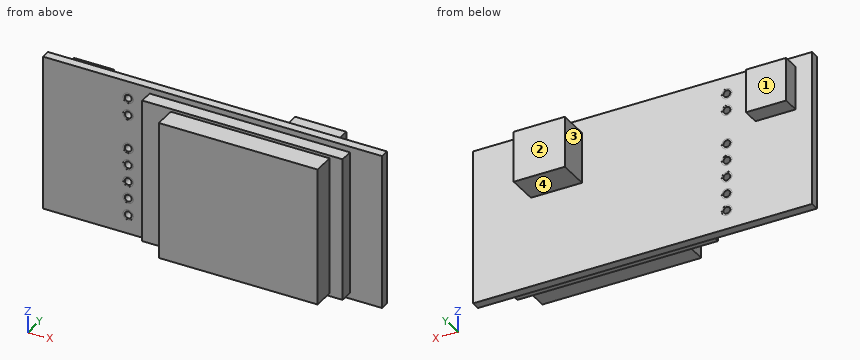
from build123d import *

# Parameters (mm, degrees)
SKETCH1_W           = 49.75
SKETCH1_H           = 22.8
BOSS_EXTRUDE1_DEPTH = 1.3
SKETCH2_W           = 7.5
SKETCH2_H           = 7.5
BOSS_EXTRUDE2_DEPTH = 4.5
SKETCH3_W           = 5.9
SKETCH3_H           = 6.4
BOSS_EXTRUDE3_DEPTH = 2.5
SKETCH4_W           = 29.4
SKETCH4_H           = 21.1
BOSS_EXTRUDE4_DEPTH = 1.95
SKETCH5_W           = 23.3
SKETCH5_H           = 20.25
BOSS_EXTRUDE5_DEPTH = 3.15
CUT_EXTRUDE1_REACH  = 29.971
SKETCH6_R           = 0.5
SKETCH7_R           = 0.75
CUT_EXTRUDE2_DEPTH  = 0.01
CUT_EXTRUDE3_START  = -0.01
SKETCH8_R           = 0.75
CUT_EXTRUDE3_DEPTH  = 0.01


with BuildPart() as part:
    # Sketch1 → Boss-Extrude1 (new body)
    with BuildSketch(Plane(origin=(0, 0, 0), x_dir=(1, 0, 0), z_dir=(0, 1, 0))):
        Rectangle(SKETCH1_W, SKETCH1_H)
    extrude(amount=BOSS_EXTRUDE1_DEPTH)

    # Sketch2 → Boss-Extrude2 (add)
    with BuildSketch(Plane(origin=(0, 1.3, 0), x_dir=(1, 0, 0), z_dir=(0, 1, 0))):
        with Locations((12.625, -5.65)):
            Rectangle(SKETCH2_W, SKETCH2_H)
    extrude(amount=BOSS_EXTRUDE2_DEPTH)

    # Sketch3 → Boss-Extrude3 (add)
    with BuildSketch(Plane(origin=(0, 1.3, 0), x_dir=(1, 0, 0), z_dir=(0, 1, 0))):
        with Locations((-19.525, -6.7)):
            Rectangle(SKETCH3_W, SKETCH3_H)
    extrude(amount=BOSS_EXTRUDE3_DEPTH)

    # Sketch4 → Boss-Extrude4 (add)
    with BuildSketch(Plane.XZ):
        with Locations((5.475, 0)):
            Rectangle(SKETCH4_W, SKETCH4_H)
    extrude(amount=BOSS_EXTRUDE4_DEPTH)

    # Sketch5 → Boss-Extrude5 (add)
    with BuildSketch(Plane.XZ.offset(1.95)):
        with Locations((6.625, 0)):
            Rectangle(SKETCH5_W, SKETCH5_H)
    extrude(amount=BOSS_EXTRUDE5_DEPTH)

    # Sketch6 → Cut-Extrude1 (cut, up to next)
    with BuildSketch(Plane.XZ, mode=Mode.PRIVATE) as cut_extrude1_sk1:
        with Locations(Location((-12.375, 8.9, 0), (0, 0, 270))):
            Circle(SKETCH6_R)
    cut_extrude1_tool1 = extrude(cut_extrude1_sk1.sketch, amount=-CUT_EXTRUDE1_REACH, mode=Mode.PRIVATE) & part.part
    # Sketch6 → Cut-Extrude1 (cut, up to next)
    with BuildSketch(Plane.XZ, mode=Mode.PRIVATE) as cut_extrude1_sk2:
        with Locations(Location((-12.375, 6.4, 0), (0, 0, 270))):
            Circle(SKETCH6_R)
    cut_extrude1_tool2 = extrude(cut_extrude1_sk2.sketch, amount=-CUT_EXTRUDE1_REACH, mode=Mode.PRIVATE) & part.part
    # Sketch6 → Cut-Extrude1 (cut, up to next)
    with BuildSketch(Plane.XZ, mode=Mode.PRIVATE) as cut_extrude1_sk3:
        with Locations(Location((-12.375, 1.4, 0), (0, 0, 270))):
            Circle(SKETCH6_R)
    cut_extrude1_tool3 = extrude(cut_extrude1_sk3.sketch, amount=-CUT_EXTRUDE1_REACH, mode=Mode.PRIVATE) & part.part
    # Sketch6 → Cut-Extrude1 (cut, up to next)
    with BuildSketch(Plane.XZ, mode=Mode.PRIVATE) as cut_extrude1_sk4:
        with Locations(Location((-12.375, -1.1, 0), (0, 0, 270))):
            Circle(SKETCH6_R)
    cut_extrude1_tool4 = extrude(cut_extrude1_sk4.sketch, amount=-CUT_EXTRUDE1_REACH, mode=Mode.PRIVATE) & part.part
    # Sketch6 → Cut-Extrude1 (cut, up to next)
    with BuildSketch(Plane.XZ, mode=Mode.PRIVATE) as cut_extrude1_sk5:
        with Locations(Location((-12.375, -3.6, 0), (0, 0, 270))):
            Circle(SKETCH6_R)
    cut_extrude1_tool5 = extrude(cut_extrude1_sk5.sketch, amount=-CUT_EXTRUDE1_REACH, mode=Mode.PRIVATE) & part.part
    # Sketch6 → Cut-Extrude1 (cut, up to next)
    with BuildSketch(Plane.XZ, mode=Mode.PRIVATE) as cut_extrude1_sk6:
        with Locations(Location((-12.375, -6.1, 0), (0, 0, 270))):
            Circle(SKETCH6_R)
    cut_extrude1_tool6 = extrude(cut_extrude1_sk6.sketch, amount=-CUT_EXTRUDE1_REACH, mode=Mode.PRIVATE) & part.part
    # Sketch6 → Cut-Extrude1 (cut, up to next)
    with BuildSketch(Plane.XZ, mode=Mode.PRIVATE) as cut_extrude1_sk7:
        with Locations(Location((-12.375, -8.6, 0), (0, 0, 270))):
            Circle(SKETCH6_R)
    cut_extrude1_tool7 = extrude(cut_extrude1_sk7.sketch, amount=-CUT_EXTRUDE1_REACH, mode=Mode.PRIVATE) & part.part
    add(cut_extrude1_tool1.solids().sort_by_distance((-12.375, 0, 8.9))[0], mode=Mode.SUBTRACT)
    add(cut_extrude1_tool2.solids().sort_by_distance((-12.375, 0, 6.4))[0], mode=Mode.SUBTRACT)
    add(cut_extrude1_tool3.solids().sort_by_distance((-12.375, 0, 1.4))[0], mode=Mode.SUBTRACT)
    add(cut_extrude1_tool4.solids().sort_by_distance((-12.375, 0, -1.1))[0], mode=Mode.SUBTRACT)
    add(cut_extrude1_tool5.solids().sort_by_distance((-12.375, 0, -3.6))[0], mode=Mode.SUBTRACT)
    add(cut_extrude1_tool6.solids().sort_by_distance((-12.375, 0, -6.1))[0], mode=Mode.SUBTRACT)
    add(cut_extrude1_tool7.solids().sort_by_distance((-12.375, 0, -8.6))[0], mode=Mode.SUBTRACT)

    # Sketch7 → Cut-Extrude2 (cut)
    with BuildSketch(Plane.XZ):
        with Locations(Location((-12.375, 8.9, 0), (0, 0, 270))):
            Circle(SKETCH7_R)
        with Locations(Location((-12.375, 6.4, 0), (0, 0, 270))):
            Circle(SKETCH7_R)
        with Locations(Location((-12.375, 1.4, 0), (0, 0, 270))):
            Circle(SKETCH7_R)
        with Locations(Location((-12.375, -1.1, 0), (0, 0, 270))):
            Circle(SKETCH7_R)
        with Locations(Location((-12.375, -3.6, 0), (0, 0, 270))):
            Circle(SKETCH7_R)
        with Locations(Location((-12.375, -6.1, 0), (0, 0, 270))):
            Circle(SKETCH7_R)
        with Locations(Location((-12.375, -8.6, 0), (0, 0, 270))):
            Circle(SKETCH7_R)
    extrude(amount=-CUT_EXTRUDE2_DEPTH, mode=Mode.SUBTRACT)

    # Sketch8 → Cut-Extrude3 (cut)
    with BuildSketch(Plane(origin=(0, 1.3, 0), x_dir=(1, 0, 0), z_dir=(0, 1, 0)).offset(CUT_EXTRUDE3_START)):
        with Locations(Location((-12.375, 8.6, 0), (0, 0, 90))):
            Circle(SKETCH8_R)
        with Locations(Location((-12.375, 6.1, 0), (0, 0, 90))):
            Circle(SKETCH8_R)
        with Locations(Location((-12.375, 3.6, 0), (0, 0, 90))):
            Circle(SKETCH8_R)
        with Locations(Location((-12.375, 1.1, 0), (0, 0, 90))):
            Circle(SKETCH8_R)
        with Locations(Location((-12.375, -1.4, 0), (0, 0, 90))):
            Circle(SKETCH8_R)
        with Locations(Location((-12.375, -6.4, 0), (0, 0, 90))):
            Circle(SKETCH8_R)
        with Locations(Location((-12.375, -8.9, 0), (0, 0, 90))):
            Circle(SKETCH8_R)
    extrude(amount=CUT_EXTRUDE3_DEPTH, mode=Mode.SUBTRACT)


solid = part.part
Geometry: final body of the model. Coordinates: model frame, mm. Face numbers are marked on the shaded views. A direction names the side the tool comes from. Give positions to 0.01 mm unless a question says otherwise; leave off trailing zeros. Write each loop counter-clockwise with the first axis right and the second up, starting at its lowest first coordinate (ties: lowest second). Pieces come first, ordered by that corner, then holes.
(1) Cut plane B-B, the plane y = 3.25. Return loops of the section in (x, z) (3 decimals), then the cut area to 3 significant figures.
(2) First-contact query: P1, Ø1.4, axis at x = -12.375, z = -1.1, coming from the +Y side; P2, Ø0.8, axis at x = -12, z = -6, coming from the -Y side; P3, Ø0.6, axis at y = -1, z = 0, coming from the +X side (3 decimals); P4, Ø0.9, axis at x = -12.375, z = 8.9, coming from the -Y side. Flat tips, straight axial feed; report the tip coordinate or a pass-through.
(3) Cut plane D-D, the plane y = -3.5. Return loops of the section in (x, z) (3 decimals), then the cut area to 3 significant figures.
(4) Ray query, line 1 (X direction, y = 1.5, z = 5.5) (3 decimals); line 2 (X direction, y = 0.45, z = 1.4) (3 decimals); line 3 (Z direction, x = 4, y = -1.25). Return the intervals inside material, ascending.
(5) Cut plane A-A, the plane z = -3.6. Return loops of the section in (x, y) (3 decimals).
(6) Mould query, pull axis X, two halves, no side actions, for the marked faces 3 and 4. Classes: released by +X, released by -X, zero draft, split by the parting line, or undercut.
(7) Access query for the marked faces 1 and 2. Directions: +Z, -Z, +X, -X, +Y, -Y. A direction counts if a zero-diameter tool reaches every point of the face in a straight line with its end or side. Return the directions, or none.
Values follow:
1. outline: (-22.475, 3.5) - (-16.575, 3.5) - (-16.575, 9.9) - (-22.475, 9.9) - close; (8.875, 1.9) - (16.375, 1.9) - (16.375, 9.4) - (8.875, 9.4) - close
1. area: 94.0 mm2
2. P1: stops at y = 1.29
2. P2: stops at y = 0
2. P3: stops at x = 20.175
2. P4: passes through
3. outline: (-5.025, -10.125) - (18.275, -10.125) - (18.275, 10.125) - (-5.025, 10.125) - close
3. area: 472 mm2
4. line 1: x = -22.475 to -16.575, 8.875 to 16.375
4. line 2: x = -24.875 to -12.875, -11.875 to 24.875
4. line 3: z = -10.55 to 10.55
5. outline: (-24.875, 0) - (-13.125, 0) - (-13.125, 0.01) - (-12.875, 0.01) - (-12.875, 1.29) - (-13.125, 1.29) - (-13.125, 1.3) - (-24.875, 1.3) - close; (-11.875, 0.01) - (-11.625, 0.01) - (-11.625, 0) - (-9.225, 0) - (-9.225, -1.95) - (-5.025, -1.95) - (-5.025, -5.1) - (18.275, -5.1) - (18.275, -1.95) - (20.175, -1.95) - (20.175, 0) - (24.875, 0) - (24.875, 1.3) - (-11.625, 1.3) - (-11.625, 1.29) - (-11.875, 1.29) - close
6. face 3: undercut
6. face 4: zero draft
7. face 1: +Z, -Z, -X, +Y
7. face 2: +Z, -Z, +X, -X, +Y
